from build123d import *

# Parameters (mm, degrees)
F1_DEPTH = 10
F2_R     = 135.50038
F3_DEPTH = 134
F4_W     = 10.05
F4_H     = 10.05
F5_DEPTH = 12.5


with BuildPart() as f1:
    # F0 (on Top) → F1 (new body)
    with BuildSketch(Plane.XY):
        with BuildLine():
            Line((-30.500877, 28.849207), (0, 0))
            Line((0, 0), (0, 58.898218))
            ThreePointArc((0, 58.898218), (-30.814656, 59.67198), (-30.500877, 28.849207))
        make_face()
        with BuildLine():
            Line((0, 58.898218), (0, 0))
            Line((0, 0), (30.500877, 28.849207))
            ThreePointArc((30.500877, 28.849207), (30.814656, 59.67198), (0, 58.898218))
        make_face()
    extrude(amount=F1_DEPTH)

    # F2 (on Front) → F3 (cut)
    with BuildSketch(Plane.XZ):
        with Locations((0, -90)):
            Circle(F2_R)
        with BuildLine():
            ThreePointArc((0, 10), (70.710678, -19.289322), (100, -90))
            ThreePointArc((100, -90), (-70.710678, -160.710678), (0, 10))
        make_face(mode=Mode.SUBTRACT)
    extrude(amount=-F3_DEPTH, mode=Mode.SUBTRACT)

    # F4 (on Top) → F5 (cut, symmetric)
    with BuildSketch(Plane.XY):
        with Locations((0, 37.200861)):
            Rectangle(F4_W, F4_H)
    extrude(amount=F5_DEPTH, both=True, mode=Mode.SUBTRACT)


solid = f1.part
Read the model definition and answer for the solid it produces. Units are mm, in the model's axes. A direction names the side the tool comes from. Give positions to 0.01 mm unless a question says otherwise; leave off trailing zeros. Write each loop counter-clockwise with the first axis right and the second up, starting at its lowest first coordinate (ties: lowest second). Pieces come first, ordered by that corner, then holes. Notation, with made-up numbers: (64, -9) - (122, -9) arc R11 cw to (122, 0) - close; hole circle Ø2 at (1.5, -2.5). An arc over 180 degrees is marked (long way). Use CSV: the item, a comma, the result in double quotes. Start each with the question number.
Item 1: The mould has two halves that part along X. Classify faces 3 (the flat face through (0, 42.226, 5)), 4 (the flat face through (-15.464, 14.627, 3.819)), 5 (the flat face through (8, 41, 0)): pulls with the +X half, pulls with the -X half, needs draft (parallel to the pull), parting line crosses it, or undercut.
Item 2: The part is cut by section C-C, the plane x = 1.5. Give the vertices of the cut face in (y, z).
Item 3: The part is cut by section D-D, the plane y = 51.5. Give the vertices of the cut face in (x, z).
Item 4: Flat-ended cylindrical pins translate along their axes: P1, Ø5, axis at x = -17, y = 38, coming from the +Z side; P2, Ø5, axis at y = 26, z = 4.5, coming from the -X side; P3, Ø3, axis at x = -3.5, z = 6.5, coming from the -Y side. Find the tip coordinate at first contact, or state that the pin passes through.
Item 5: The part is cut by section A-A, the plane y = 34. Give the vertices of the cut face in (x, z) (3 decimals), and give its area (3 significant figures).
Item 6: For faces 1 (the flat face through (5.025, 37, 5)), 2 (the flat face through (15.037, 14.223, 3.819)), determine the directions among +Z, -Z, +X, -X, +Y, -Y from which every point of the face is accessible in a straight line to the end or side of a thin tool.
Item 7: Consider line 1 (Z direction, x = -5, y = 54); line 2 (Y direction, x = 2, z = 8.5); line 3 (Y direction, x = -3, z = 9.75). Determine where each line is inside the solid, lowest interval first.
Taken from the geometry:
1,face 3,"undercut"
1,face 4,"pulls with the -X half"
1,face 5,"needs draft"
2,outline,"(1.42, 0) - (32.18, 0) - (32.18, 9.99) - (1.42, 9.99) - close; (42.23, 0) - (60.38, 0) - (60.38, 9.99) - (42.23, 9.99) - close"
3,outline,"(-36, 0) - (36, 0) - (36, 3.3) arc R100 ccw to (-36, 3.3) - close"
4,P1,"z = 8.94"
4,P2,"x = -30.13"
4,P3,"y = 1.89"
5,outline,"(-34.502, 0) - (-5.025, 0) - (-5.025, 9.874) arc R100 ccw to (-34.502, 3.86) - close; (5.025, 0) - (34.502, 0) - (34.502, 3.86) arc R100 ccw to (5.025, 9.874) - close"
5,area,"451 mm2"
6,face 1,"+Z, -Z"
6,face 2,"+Z, -Z, +X, -Y"
7,line 1,"0 to 9.87"
7,line 2,"1.89 to 32.18, 42.23 to 60.81"
7,line 3,"2.84 to 32.18, 42.23 to 61.6"
